from build123d import *

# Parameters (mm, degrees)
F0_R     = 70.1167257922
F1_DEPTH = 25.4
F2_DEPTH = 9.525
F0_W     = 114.0985068913
F0_H     = 56.9764161581
F0_R_2   = 17.4384026712
F3_DEPTH = 3.175
F5_DEPTH = 6.35


with BuildPart() as f1:
    # F0 (on Top) → F1 (new body)
    with BuildSketch(Plane.XY):
        Circle(F0_R)
        with BuildLine():
            ThreePointArc((57.0492534457, 28.4882080791), (62.0646413805, 14.6347397849), (63.7667257922, 0))
            ThreePointArc((63.7667257922, 0), (62.0646413805, -14.6347397849), (57.0492534457, -28.4882080791))
            ThreePointArc((57.0492534457, -28.4882080791), (0, -63.7667257922), (-57.0492534457, -28.4882080791))
            ThreePointArc((-57.0492534457, -28.4882080791), (-63.7667257922, 0), (-57.0492534457, 28.4882080791))
            ThreePointArc((-57.0492534457, 28.4882080791), (0, 63.7667257922), (57.0492534457, 28.4882080791))
        make_face(mode=Mode.SUBTRACT)
    extrude(amount=F1_DEPTH)

    # F0 (on Top) → F2 (join)
    with BuildSketch(Plane.XY):
        with BuildLine():
            Line((-57.0492534457, 28.4882080791), (57.0492534457, 28.4882080791))
            ThreePointArc((57.0492534457, 28.4882080791), (0, 63.7667257922), (-57.0492534457, 28.4882080791))
        make_face()
        with BuildLine():
            Line((-57.0492534457, -28.4882080791), (-57.0492534457, 28.4882080791))
            ThreePointArc((-57.0492534457, 28.4882080791), (-63.7667257922, 0), (-57.0492534457, -28.4882080791))
        make_face()
        with BuildLine():
            ThreePointArc((-57.0492534457, -28.4882080791), (0, -63.7667257922), (57.0492534457, -28.4882080791))
            Line((57.0492534457, -28.4882080791), (-57.0492534457, -28.4882080791))
        make_face()
        with BuildLine():
            ThreePointArc((57.0492534457, -28.4882080791), (62.0646413805, -14.6347397849), (63.7667257922, 0))
            ThreePointArc((63.7667257922, 0), (62.0646413805, 14.6347397849), (57.0492534457, 28.4882080791))
            Line((57.0492534457, 28.4882080791), (57.0492534457, -28.4882080791))
        make_face()
    extrude(amount=F2_DEPTH)

    # F0 (on Top) → F3 (join)
    with BuildSketch(Plane.XY):
        Rectangle(F0_W, F0_H)
        with Locations((-31.0109015554, 0)):
            Circle(F0_R_2, mode=Mode.SUBTRACT)
        with Locations((31.0109015554, 0)):
            Circle(F0_R_2, mode=Mode.SUBTRACT)
    extrude(amount=F3_DEPTH)

    # F4 (on face) → F5 (cut)
    with BuildSketch(Plane.XY.offset(9.525)):
        with BuildLine():
            Line((-8.9004095644, 63.1425215512), (-8.9004095644, 28.4882080791))
            Line((-8.9004095644, 28.4882080791), (8.2985507539, 28.4882080791))
            Line((8.2985507539, 28.4882080791), (8.2985507539, 63.224436523))
            ThreePointArc((8.2985507539, 63.224436523), (-0.3037038403, 63.7660025581), (-8.9004095644, 63.1425215512))
        make_face()
    extrude(amount=-F5_DEPTH, mode=Mode.SUBTRACT)


solid = f1.part
Can you work these out from the model? Positions are in its coordinate system, mm. A direction names the side the tool comes from. Coordinates: 2 decimals unless noted, no trailing zeros. Loops run counter-clockwise (first coordinate to the right, second up) from the corner with the lowest first, then second, coordinate; pieces in that order, holes last. Notation, with made-up numbers: M 9,6 L 37,6 A29 cw 37,34 Z; hole C -7.5,7.25 d5. An arc over 180 degrees is marked long. Return JSON: item names as keys, results as strings. Group by question number.
Item 1: Imagine slicing it at A-A (z = 6.75). Please give me the cut outline in (x, y).
Item 2: If I drill on L1, parallel to Z at x = -54.5, y = -18 (3 decimals); L2, parallel to X at y = 30, z = 22; L3, parallel to Y at x = 9.5, z = 6, over which ranges is the centre line in solid material (lowest first)? Write a range as from..to.
Item 3: On a 3-axis mill with a long thin cutter (end or side, diameter ignored), from which of +Z, -Z, +X, -X, +Y, -Y can I reach the whole of each face in a straight line? I mean faces 4 (the flat face through (32, 28.488, 6)), 5 (the cylindrical face through (-43.86, 11.79, 1.57)). Say none if no direction works.
Item 4: Imagine slicing it at C-C (y = -3.5). Please give me the cut outline in (x, z) (3 decimals).
Item 5: Thinking about a two-plate mould opening in Y: for faces 1 (the cylindrical face through (37.694, 59.123, 12.522)), 2 (the flat face through (-16, -62, 25.4)), 3 (the flat face through (-60, 0, 9.525)), which applies, released by +Y, released by -Y, zero draft, split by the parting line, or undercut?
Item 6: Imagine slicing it at B-B (x = 0). Please give me the cut outline in (y, z) (3 decimals), and give its area (3 significant figures).
Item 7: Imagine slicing it at D-D (x = 46). Please give me the cut outline in (y, z) (3 decimals), and give its area (3 significant figures).
Item 8: I'm going to push flat-ended pins straight in: pin 1 Ø6 at (x, y) = (45, 40) entering from +Z (3 decimals); pin 2 Ø5 at (x, z) = (-36, 5.5) entering from -Y; pin 3 Ø1.9 at (y, z) = (49, 6) entering from +X. Where does each tip first touch, or does it pass through?
Verdict:
{
 "1": {"outline": "C 0,0 d140.23; hole M -57.05,-28.49 L 57.05,-28.49 L 57.05,28.49 L 8.3,28.49 L 8.3,63.22 A63.77 ccw -8.9,63.14 L -8.9,28.49 L -57.05,28.49 Z"},
 "2": {"L1": "z = 0..3.175", "L2": "x = -63.37..-56.27, 56.27..63.37", "L3": "y = -69.47..-28.49, 28.49..69.47"},
 "3": {"face 4": "+Z", "face 5": "+Z, -Z"},
 "4": {"outline": "M -70.029,0 L -48.094,0 L -48.094,3.175 L -57.049,3.175 L -57.049,9.525 L -63.671,9.525 L -63.671,25.4 L -70.029,25.4 Z; M -13.927,0 L 13.927,0 L 13.927,3.175 L -13.927,3.175 Z; M 48.094,0 L 70.029,0 L 70.029,25.4 L 63.671,25.4 L 63.671,9.525 L 57.049,9.525 L 57.049,3.175 L 48.094,3.175 Z"},
 "5": {"face 1": "split by the parting line", "face 2": "zero draft", "face 3": "undercut"},
 "6": {"outline": "M -70.117,0 L 70.117,0 L 70.117,25.4 L 63.767,25.4 L 63.767,3.175 L -28.488,3.175 L -28.488,9.525 L -63.767,9.525 L -63.767,25.4 L -70.117,25.4 Z", "area": "952 mm^2"},
 "7": {"outline": "M -52.918,0 L -8.912,0 L -8.912,3.175 L -28.488,3.175 L -28.488,9.525 L -44.161,9.525 L -44.161,25.4 L -52.918,25.4 Z; M 8.912,0 L 52.918,0 L 52.918,25.4 L 44.161,25.4 L 44.161,9.525 L 28.488,9.525 L 28.488,3.175 L 8.912,3.175 Z", "area": "868 mm^2"},
 "8": {"pin 1": "stops at z = 9.525", "pin 2": "stops at y = -61.6", "pin 3": "stops at x = 51.06"}
}
